Autodesk Inventor part; units mm, degrees
ref_plane "YZ Plane" through (0, 0, 0) normal (1, 0, 0) x (0, 1, 0)
ref_plane "XZ Plane" through (0, 0, 0) normal (0, 1, 0) x (-1, 0, 0)
ref_plane "XY Plane" through (0, 0, 0) normal (0, 0, 1) x (1, 0, 0)
sketch "Sketch6" plane through (0, 0, 0) normal (0, 1, 0) x (-1, 0, 0)
  line L0 (0, 0) -> (4, 0)
  line L1 (4, 0) -> (4, -15)
  line L2 (4, -15) -> (0, -15)
  line L3 (0, -15) -> (0, 0)
  dimension "d17" = 4
  dimension "d18" = 15
extrude "Extrusion5" add sketch "Sketch6" along normal blind 4
sketch "Sketch7" plane through (-4, 0, 0) normal (0, 0, 1) x (1, 0, 0)
  line L0 (0, 0) -> (0, 4)
  line L1 (4, 0) -> (4, 4)
  line L2 (0, 3.25) -> (4, 3.25)
  line L3 (4, 3.25) -> (4, 0.75)
  line L4 (4, 0.75) -> (0, 0.75)
  line L5 (0, 0.75) -> (0, 3.25)
  line L6 (0, 4) -> (4, 4)
  line L7 (4, 0) -> (0, 0)
  dimension "d21" = 0.75
  dimension "d22" = 0.75
extrude "Extrusion6" cut sketch "Sketch7" against normal blind 6 contours L0 L2 L1 L4
sketch "Sketch8" plane through (0, 4, 0) normal (0, 1, 0) x (1, 0, 0)
  line L0 (-4, 6) -> (0, 6)
  line L1 (-4, 15) -> (-4, 0)
  line L2 (0, 0) -> (-4, 0)
  line L3 (-4, 6) -> (-4, 0)
  circle A0 centre (-2, 2) radius 1
  dimension "d25" = 2
extrude "Extrusion7" cut sketch "Sketch8" against normal blind 4
sketch "Sketch9" plane through (0, 0, -15) normal (0, 0, -1) x (-1, 0, 0)
  line L0 (4, 0) -> (0, 0)
  line L1 (4, 0) -> (4, 4)
  line L2 (0, 4) -> (4, 4)
  line L3 (0, 0) -> (0, 4)
  circle A0 centre (2, 2) radius 1
  point P0 (0, 0)
  dimension "d28" = 2
extrude "Extrusion8" cut sketch "Sketch9" against normal blind 8 contours A0
sketch "Sketch10" plane through (0, 0, 0) normal (1, 0, 0) x (0, 0, -1)
  line L0 (0, 3.25) -> (6, 3.25)
  line L1 (6, 3.25) -> (6, 0.75)
  line L2 (6, 0.75) -> (0, 0.75)
  line L3 (0, 0) -> (0, 0.75)
  line L4 (15, 0) -> (0, 0)
  line L5 (15, 0) -> (15, 4)
  line L6 (0, 4) -> (15, 4)
  line L7 (0, 3.25) -> (0, 4)
  line L8 (15, 4) -> (0, 4)
  line L9 (4, 4) -> (7.2907, 4) construction
  line L10 (15, 0) -> (15, 4)
  line L11 (7.2907, 4) -> (15, 3.25) construction
  spline S0 degree 2 poles (4, 4) (7.2907, 4) (15, 3.25) knots 1 1 1 2 2 2
  line L12 (6, 3.25) -> (6, 0.75)
  line L13 (6, 2) -> (3.448, 2)
  line L14 (4, 0) -> (7.2907, 0) construction
  line L15 (7.2907, 0) -> (15, 0.75) construction
  spline S1 degree 2 poles (4, 0) (7.2907, 0) (15, 0.75) knots 1 1 1 2 2 2
  dimension "d31" = 0.75
extrude "Extrusion9" cut sketch "Sketch10" against normal blind 8 contours L6 L5 S0
pattern_circular "Circular Pattern1" count 2 over 360 about axis through (-2, 2, -15) along (0, 0, 1) of "Extrusion9"
fillet "Fillet1" radius 2 4 edges at (0, 3.625, 0) (-4, 3.625, 0) (0, 0.375, 0) (-4, 0.375, 0)
chamfer "Chamfer1" distance 8 distance2 0.5 1 edges at (0, 2, -15) measured on face at (0, 1.5833, -12)
chamfer "Chamfer2" distance 0.5 distance2 8 1 edges at (-4, 2, -15) measured on face at (-3.6667, 2, -15)
properties part number "metalClevisis" material "Aluminum 6061"
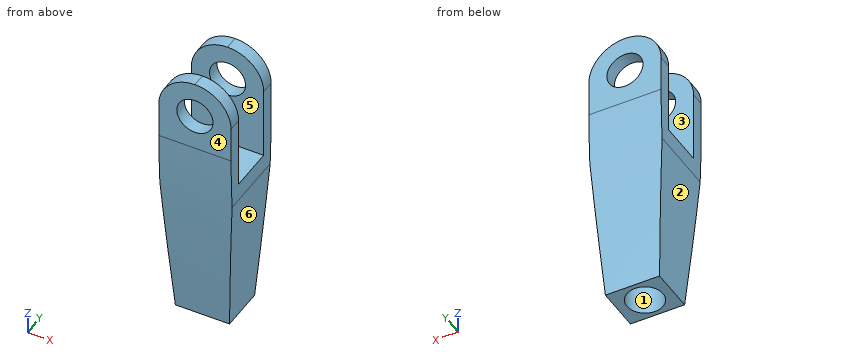
Part model, mm, in its own coordinate system. Face numbers are marked on the shaded views. A direction names the side the tool comes from. Give positions to 0.01 mm unless a question says otherwise; leave off trailing zeros. Loops run counter-clockwise (first coordinate to the right, second up) from the corner with the lowest first, then second, coordinate; pieces in that order, holes last.
(1) Band-saw the part on B-B (y = 2). Write the cut outline in (x, z).
Return value:
outline: (-4, -7) - (-3.5, -15) - (-3, -15) - (-3, -7) - (-1, -7) - (-1, -15) - (-0.5, -15) - (0, -7) - (0, -6) - (-4, -6) - close
(2) Pull direction Y, two halves, no side cores. Call the marked faces 4, 5 and 6: pulls with the +Y half, pulls with the -Y half, needs draft (parallel to the pull), parting line crosses it, or undercut.
Return value:
face 4: pulls with the -Y half
face 5: undercut
face 6: needs draft
(3) Band-saw the part on A-A (z = -1.5). Write the cut outline in (x, y), and give its area (3 significant figures).
Return value:
outline: (-3.94, 0) - (-2.87, 0) - (-2.87, 0.75) - (-3.94, 0.75) - close; (-3.94, 3.25) - (-2.87, 3.25) - (-2.87, 4) - (-3.94, 4) - close; (-1.13, 0) - (-0.06, 0) - (-0.06, 0.75) - (-1.13, 0.75) - close; (-1.13, 3.25) - (-0.06, 3.25) - (-0.06, 4) - (-1.13, 4) - close
area: 3.21 mm2
(4) Drill centre lines: line 1 along Y through (x, z) = (-1.05, -4); line 2 along X through (y, z) = (3.8, -2); line 3 along Y through (x, z) = (-2.25, -8). Where is each one in solid material? Low to high.
Return value:
line 1: y = 0 to 0.75, 3.25 to 4
line 2: x = -4 to -3, -1 to 0
line 3: y = 0.16 to 1.03, 2.97 to 3.84
(5) Pin check, flat tips, straight feed: pin 1 (1 mm diameter, centred on y = 3.5, z = -11.5, fed in from +X); pin 2 (2 mm diameter, centred on x = -2.5, z = -3.5, fed in from -Y). Stop position of each tip, or through.
Return value:
pin 1: stops at x = -0.25
pin 2: stops at y = 0
(6) 3-axis set-ups, long thin cutter, end or side, ignore diameter. For the marked faces 1, 2 and 3: which of +Z, -Z, +X, -X, +Y, -Y reach the whole face in a straight line?
Return value:
face 1: -Z
face 2: -Z, -X, +Y, -Y
face 3: +Z, +X, -X
(7) Band-saw the part on C-C (x = -2.2). Count the separate pieces of the cut face and the enclosed holes in it, and give its area (3 significant figures).
Return value:
separate pieces: 3
enclosed holes: 0
area: 19.8 mm2
